Here's how the part is built. I have some questions about the finished solid (model axes, mm). Face numbers are marked on the shaded views. Round coordinates to 2 decimals unless told otherwise and drop trailing zeros. Loops run counter-clockwise (first coordinate to the right, second up) from the corner with the lowest first, then second, coordinate; pieces in that order, holes last. Notation, with made-up numbers: (71, -15) - (103, -15) arc R15 cw to (103, 10) - close; hole circle Ø1 at (5, 56). An arc over 180 degrees is marked (long way). Answer as a JSON object with one key per item and string values. Group by question number.
1) I want a section at B-B, the plane x = 9.5. Please give me the cut outline in (y, z).
2) If I drill on line 1 along Z through (x, y) = (9.5, -8.95); line 2 along Z through (x, y) = (44, 1.25); line 3 along Z through (x, y) = (9.5, -9.1), over which ranges is the centre line in solid material (lowest first)? Write a range as [from, to].
3) I want a section at C-C, the plane x = 109.5. Please give me the cut outline in (y, z), then the cut area to 3 significant figures.
4) I want a section at A-A, the plane z = 9.5. Please give me the cut outline in (x, y).
5) Will these pins go through, and if not, where does the flat tip stop? P1, Ø4, axis at x = 134.5, z = 114.5, coming from the +Y side; P2, Ø1.5, axis at y = 2, z = 55, coming from the +X side; P3, Ø5, axis at y = 5, z = 47, coming from the +X side.
6) If we mould it in two halves opening along Z, with no side actions, what happens to the marked faces 1, 2 and 3? For each: pulls with the +Z half, pulls with the -Z half, needs draft (parallel to the pull), parting line crosses it, or undercut.
7) I want a section at D-D, the plane z = 62. Please give me the cut outline in (x, y), then the cut area to 3 significant figures.
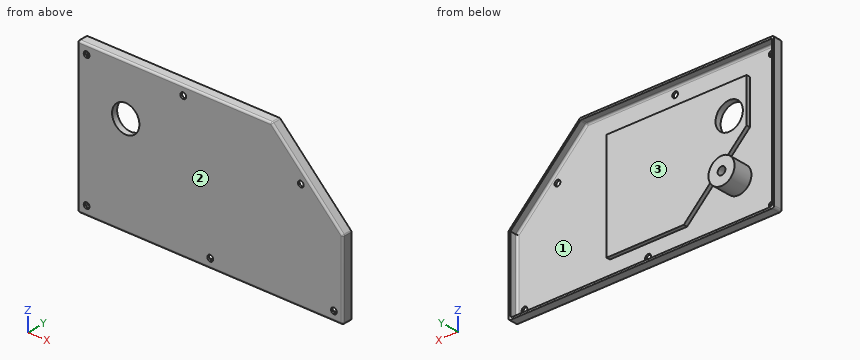
from build123d import *

# Parameters (mm, degrees)
F1_DEPTH  = 10
F2_T      = -2
F4_DEPTH  = 4
F5_R      = 13.5
F6_DEPTH  = 20
F7_R      = 4
F8_DEPTH  = 20
F10_D     = 6
F11_R     = 2
F12_R     = 2
F13_R     = 14.15
F14_DEPTH = 6.001


with BuildPart() as f1:
    # F0 (on Front) → F1 (new body)
    with BuildSketch(Plane.XZ):
        Polygon((0, 154), (0, 0), (275, 0), (275, 80), (201, 154), align=None)
    extrude(amount=F1_DEPTH)

    # F2
    f2_openings = [f1.faces().sort_by_distance(p)[0] for p in [
        (129.700907, 0, 73.382695),
    ]]
    offset(amount=F2_T, openings=f2_openings)

    # F3 (on face) → F4 (join)
    with BuildSketch(Plane(origin=(0, -8, 0), x_dir=(-1, 0, 0), z_dir=(0, 1, 0))):
        Polygon((-32, 87), (-32, 132), (-177, 132), (-177, 22), (-97, 22), align=None)
    extrude(amount=F4_DEPTH)

    # F5 (on face) → F6 (join)
    with BuildSketch(Plane(origin=(0, -8, 0), x_dir=(-1, 0, 0), z_dir=(0, 1, 0))):
        with Locations((-44, 44)):
            Circle(F5_R)
    extrude(amount=F6_DEPTH)

    # F7 (on face) → F8 (cut, through all)
    with BuildSketch(Plane(origin=(0, 12, 0), x_dir=(-1, 0, 0), z_dir=(0, 1, 0))):
        with Locations((-44, 44)):
            Circle(F7_R)
    extrude(amount=-F8_DEPTH, mode=Mode.SUBTRACT)

    # F10 (through all)
    with Locations(Plane.XZ.offset(10)):
        with Locations((9.5, 144.5), (109.5, 144.5), (231.2824855787, 110.2824855787), (265.5, 9.5), (137.5, 9.5), (9.5, 9.5)):
            Hole(F10_D / 2)

    # F11
    f11_edges = [f1.edges().sort_by_distance(p)[0] for p in [
        (0, -10, 77),
        (137.5, -10, 0),
        (238, -10, 117),
        (275, -10, 40),
        (275, -5, 0),
        (275, -5, 80),
        (201, -5, 154),
        (0, -5, 0),
        (100.5, -10, 154),
        (0, -5, 154),
    ]]
    fillet(f11_edges, radius=F11_R)

    # F12
    f12_edges = [f1.edges().sort_by_distance(p)[0] for p in [
        (273, -4, 2),
        (137.5, -8, 2),
        (273, -8, 40.585786),
        (236.585786, -8, 115.585786),
        (200.171573, -4, 152),
        (101.085786, -8, 152),
        (2, -4, 2),
        (2, -8, 77),
    ]]
    fillet(f12_edges, radius=F12_R)

    # F13 (on face) → F14 (cut, through all)
    with BuildSketch(Plane(origin=(0, -4, 0), x_dir=(-1, 0, 0), z_dir=(0, 1, 0))):
        with Locations((-50, 102)):
            Circle(F13_R)
    extrude(amount=-F14_DEPTH, mode=Mode.SUBTRACT)


solid = f1.part
Outcome:
{
 "1": {"outline": "(-10, 2) arc R2 ccw to (-8, 0) - (0, 0) - (0, 2) - (-6, 2) arc R2 cw to (-8, 4) - (-8, 6.5) - (-10, 6.5) - close; (-10, 12.5) - (-8, 12.5) - (-8, 141.5) - (-10, 141.5) - close; (-10, 147.5) - (-8, 147.5) - (-8, 150) arc R2 cw to (-6, 152) - (0, 152) - (0, 154) - (-8, 154) arc R2 ccw to (-10, 152) - close"},
 "2": {"line 1": "[0.24, 6.5], [12.5, 141.5], [147.5, 153.76]", "line 2": "[30.5, 40], [48, 57.5]", "line 3": "[0.33, 6.5], [12.5, 141.5], [147.5, 153.67]"},
 "3": {"outline": "(-10, 2) arc R2 ccw to (-8, 0) - (0, 0) - (0, 2) - (-6, 2) arc R2 cw to (-8, 4) - (-8, 22) - (-4, 22) - (-4, 132) - (-8, 132) - (-8, 141.5) - (-10, 141.5) - close; (-10, 147.5) - (-8, 147.5) - (-8, 150) arc R2 cw to (-6, 152) - (0, 152) - (0, 154) - (-8, 154) arc R2 ccw to (-10, 152) - close", "area": "768 mm^2"},
 "4": {"outline": "(0, -8) arc R2 ccw to (2, -10) - (6.5, -10) - (6.5, -8) - (4, -8) arc R2 cw to (2, -6) - (2, 0) - (0, 0) - close; (12.5, -10) - (134.5, -10) - (134.5, -8) - (12.5, -8) - close; (140.5, -10) - (262.5, -10) - (262.5, -8) - (140.5, -8) - close; (268.5, -10) - (273, -10) arc R2 ccw to (275, -8) - (275, 0) - (273, 0) - (273, -6) arc R2 cw to (271, -8) - (268.5, -8) - close"},
 "5": {"P1": "y = -4", "P2": "x = 52.79", "P3": "x = 57.49"},
 "6": {"face 1": "undercut", "face 2": "needs draft", "face 3": "undercut"},
 "7": {"outline": "(0, -8) arc R2 ccw to (2, -10) - (273, -10) arc R2 ccw to (275, -8) - (275, 0) - (273, 0) - (273, -6) arc R2 cw to (271, -8) - (177, -8) - (177, -4) - (57, -4) - (57, -8) - (4, -8) arc R2 cw to (2, -6) - (2, 0) - (0, 0) - close", "area": "1,060 mm^2"}
}
